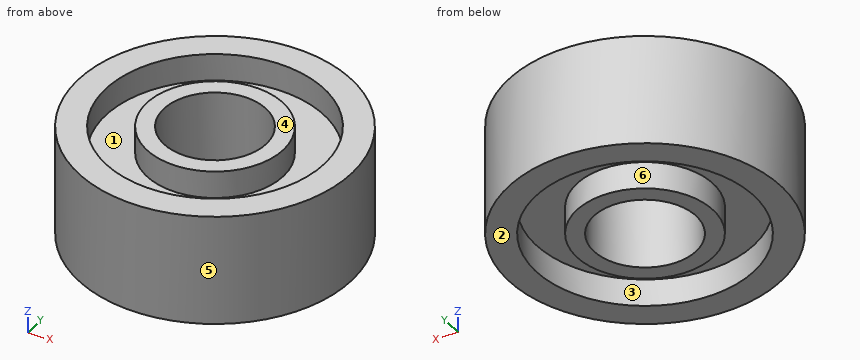
Solid Edge part; units mm, degrees
sketch "Sketch1" plane through (0, 0, 0) normal (0, 0, 1) x (1, 0, 0)
  circle A0 centre (0, 0) radius 4
  circle A1 centre (0, 0) radius 1.5
extrude "Protrusion1" add sketch "Sketch1" along normal mid plane 3.25
sketch "Sketch2" plane through (0, 0, 1.625) normal (0, 0, 1) x (1, 0, 0)
  circle A0 centre (0, 0) radius 3.2
  circle A1 centre (0, 0) radius 2
extrude "VaciadoExtruido_1" cut sketch "Sketch2" against normal blind 0.8
mirror "Mirror1" about plane through (0, 0, 0) normal (0, 0, 1) of "VaciadoExtruido_1"
Source: CAD feature listing. Evaluate the final solid. Frame: model axes, mm. Face numbers are marked on the shaded views. A direction names the side the tool comes from. Give positions to 0.01 mm unless a question says otherwise; leave off trailing zeros. Write each loop counter-clockwise with the first axis right and the second up, starting at its lowest first coordinate (ties: lowest second). Pieces come first, ordered by that corner, then holes. Notation, with made-up numbers: M 32.25,53.25 L 87.25,53.25 A26 ccw 87.25,92.25 Z; hole C 74,6.5 d8. An arc over 180 degrees is marked long. Return JSON: item names as keys, results as strings. Group by question number.
1) Draft query along X for the marked faces 4, 5 and 6. Return one class per face: released by +X, released by -X, zero draft, split by the parting line, or undercut.
2) First-contact query: pin 1 Ø2.5 at (x, y) = (0, 0) entering from -Z; pin 2 Ø1 at (y, z) = (-1.5, 1) entering from +X. Flat tips, straight axial feed; report the tip coordinate or a pass-through.
3) Cut plane A-A, the plane x = 0. Output: boundary loops of the cut face in (y, z) (3 decimals), then the cut area to 3 significant figures.
4) Cut plane D-D, the plane z = 0.6. Output: boundary loops of the cut face in (x, y), then the cut area to 3 significant figures.
5) Cut plane C-C, the plane z = -1.1. Output: boundary loops of the cut face in (x, y), then the cut area to 3 significant figures.
6) Set-up query: the marked faces 1, 2 and 3. Return all of +Z, -Z, +X, -X, +Y, -Y with unobstructed straight access to the full face (end or side cutting, diameter ignored); none if empty.
7) Ray query, L1, parallel to Y at x = 0, z = -1.15; L2, parallel to X at y = -1.75, z = -1; L3, parallel to X at y = -0.5, z = -1.15. Return the intervals inside material, ascending.
Data:
{
 "1": {"face 4": "zero draft", "face 5": "split by the parting line", "face 6": "undercut"},
 "2": {"pin 1": "passes through", "pin 2": "stops at x = 3.87"},
 "3": {"outline": "M -4,-1.625 L -3.2,-1.625 L -3.2,-0.825 L -2,-0.825 L -2,-1.625 L -1.5,-1.625 L -1.5,1.625 L -2,1.625 L -2,0.825 L -3.2,0.825 L -3.2,1.625 L -4,1.625 Z; M 1.5,-1.625 L 2,-1.625 L 2,-0.825 L 3.2,-0.825 L 3.2,-1.625 L 4,-1.625 L 4,1.625 L 3.2,1.625 L 3.2,0.825 L 2,0.825 L 2,1.625 L 1.5,1.625 Z", "area": "12.4 mm²"},
 "4": {"outline": "C 0,0 d8; hole C 0,0 d3", "area": "43.2 mm²"},
 "5": {"outline": "C 0,0 d8; C 0,0 d4; hole C 0,0 d6.4; hole C 0,0 d3", "area": "23.6 mm²"},
 "6": {"face 1": "+Z", "face 2": "-Z, +X, -X, +Y, -Y", "face 3": "-Z"},
 "7": {"L1": "y = -4 to -3.2, -2 to -1.5, 1.5 to 2, 3.2 to 4", "L2": "x = -3.6 to -2.68, -0.97 to 0.97, 2.68 to 3.6", "L3": "x = -3.97 to -3.16, -1.94 to -1.41, 1.41 to 1.94, 3.16 to 3.97"}
}
